Read the model definition and answer for the solid it produces. Units are mm, in the model's axes. A direction names the side the tool comes from. Coordinates: 2 decimals unless noted, no trailing zeros. Order: outer loops, then holes, each group sorted by start corner. A loop starts at its lowest first (then second) coordinate and runs counter-clockwise, first axis right, second up. Notation, with made-up numbers: M 74.5,44 L 103.5,44 A20 ccw 103.5,71 Z; hole C 35,72.5 d2. An arc over 180 degrees is marked long. Put each result on its own line as item: value.
from build123d import *

# Parameters (mm, degrees)
SKETCH1_R                    = 4
BASE_FLANGE1_DEPTH           = 0.8128
EDGE_FLANGE1_STRIP_W         = 4.8768
EDGE_FLANGE1_STRIP_H         = 0.8128
EDGE_FLANGE1_STRIP_CUT_DEPTH = 50
EDGE_FLANGE1_DEPTH           = 50
FILLET2_R                    = 2
F_5_0MM_DOWEL_HOLE1_D        = 5


# Sheet-metal steps are written as plain solids
with BuildPart() as part:
    # Sketch1 → Base-Flange1 (new body)
    with BuildSketch(Plane.XY):
        with BuildLine():
            Line((-25, 0), (25, 0))
            Line((25, 0), (25, 5.5))
            ThreePointArc((25, 5.5), (24.414213562, 6.914213562), (23, 7.5))
            Line((23, 7.5), (10, 7.5))
            ThreePointArc((10, 7.5), (8.585786438, 8.085786438), (8, 9.5))
            Line((8, 9.5), (8, 13.64))
            ThreePointArc((8, 13.64), (0, 21.64), (-8, 13.64))
            Line((-8, 13.64), (-8, 9.5))
            ThreePointArc((-8, 9.5), (-8.585786438, 8.085786438), (-10, 7.5))
            Line((-10, 7.5), (-23, 7.5))
            ThreePointArc((-23, 7.5), (-24.414213562, 6.914213562), (-25, 5.5))
            Line((-25, 5.5), (-25, 0))
        make_face()
        with Locations((0, 13.64)):
            Circle(SKETCH1_R, mode=Mode.SUBTRACT)
    extrude(amount=-BASE_FLANGE1_DEPTH)

    # Edge-Flange1 strip (across the edge) → Edge-Flange1 strip cut (cut)
    with BuildSketch(Plane(origin=(25, 0, -0.8128), x_dir=(0, 1, 0), z_dir=(-1, 0, 0))):
        with Locations((-1.6256, -0.4064)):
            Rectangle(EDGE_FLANGE1_STRIP_W, EDGE_FLANGE1_STRIP_H)
    extrude(amount=EDGE_FLANGE1_STRIP_CUT_DEPTH, mode=Mode.SUBTRACT)

    # Edge-Flange1 section (across the edge) → Edge-Flange1 (add)
    with BuildSketch(Plane(origin=(25, 0, -0.8128), x_dir=(0, 1, 0), z_dir=(-1, 0, 0))):
        with BuildLine():
            Line((-0.8128, 0.8128), (-0.8128, 9.1872))
            Line((-0.8128, 9.1872), (0, 9.1872))
            Line((0, 9.1872), (0, 0.8128))
            ThreePointArc((0, 0.8128), (0.238063608, 0.238063608), (0.8128, 0))
            Line((0.8128, 0), (0.8128, -0.8128))
            ThreePointArc((0.8128, -0.8128), (-0.336672783, -0.336672783), (-0.8128, 0.8128))
        make_face()
    extrude(amount=EDGE_FLANGE1_DEPTH)

    # Fillet2
    fillet2_edges = [part.edges().sort_by_distance(p)[0] for p in [
        (25, -0.4064, -10),
        (-25, -0.4064, -10),
    ]]
    fillet(fillet2_edges, radius=FILLET2_R)

    # Ø5.0mm Dowel Hole1 (through all)
    with Locations(Plane(origin=(0, 0, 0), x_dir=(1, 0, 0), z_dir=(0, 1, 0))):
        with Locations((-12.5, 5.8128), (12.5, 5.8128)):
            Hole(F_5_0MM_DOWEL_HOLE1_D / 2)


solid = part.part
Q1. A tool of negligible diameter and unlimited length cuts with its end or side. For faces 5 (the face through (-25, -0.2, -2.5)), 6 (the face through (0, 7, -0.813)), from which of +Z, -Z, +X, -X, +Y, -Y can it reach the whole face along a straight path? Write none if from no direction.
Answers below:
face 5: +Z, -Z, -X, +Y, -Y
face 6: -Z, +X, -X, +Y
Q2. Given pin 1 (2 mm diameter, centred on x = 1.5, z = -2, fed in from +Y); pin 2 (10.5 mm diameter, centred on x = 0, y = 13.64, fed in from +Z); pin 3 (10.5 mm diameter, centred on x = 1.5, y = 14, fed in from -Z); pin 4 (3 mm diameter, centred on y = 15, z = -2.5, fed in from -X), each flat-ended and moving along its own axis, determine where each tip first touches the part or whether it passes through.
Answers below:
pin 1: stops at y = 0.29
pin 2: stops at z = 0
pin 3: stops at z = -0.81
pin 4: passes through
Q3. For a pull along Y with two mould halves and no side action, classify faces 1 (the face through (0, -0.813, -6)), 2 (the face through (0, 0, -6)), 3 (the face through (-10, -0.4, -5.9)), 4 (the face through (-0.867, 9.735, -0.401)) as +Y half, -Y half, draft (parallel to the pull), parting line (faces both ways), or undercut.
Answers below:
face 1: -Y half
face 2: +Y half
face 3: draft
face 4: undercut
Q4. Find section C-C on x = -19.5. Write down the section's boundary in (y, z), plus the area to 3 significant figures.
Answers below:
outline: M -0.81,-10 L 0,-10 L 0,-1.63 A0.81 cw 0.81,-0.81 L 7.5,-0.81 L 7.5,0 L 0.81,0 A1.63 ccw -0.81,-1.63 Z
area: 13.8 mm^2
Q5. Find section B-B on z = -7.5. Write down the section's boundary in (x, y).
Answers below:
outline: M -25,-0.81 L -14.34,-0.81 L -14.34,0 L -25,0 Z; M -10.66,-0.81 L 10.66,-0.81 L 10.66,0 L -10.66,0 Z; M 14.34,-0.81 L 25,-0.81 L 25,0 L 14.34,0 Z
Q6. Consider line 1 along Y through (x, z) = (9, -5); line 2 along Y through (x, z) = (0, -0.2). Determine where each line is inside the solid, lowest interval first.
Answers below:
line 1: y = -0.81 to 0
line 2: y = 0.03 to 9.64, 17.64 to 21.64
Q7. Find section D-D on x = 0. Write down the section's boundary in (y, z), plus the area to 3 significant figures.
Answers below:
outline: M -0.81,-10 L 0,-10 L 0,-1.63 A0.81 cw 0.81,-0.81 L 9.64,-0.81 L 9.64,0 L 0.81,0 A1.63 ccw -0.81,-1.63 Z; M 17.64,-0.81 L 21.64,-0.81 L 21.64,0 L 17.64,0 Z
area: 18.8 mm^2
Q8. Find section A-A on x = -12.5. Write down the section's boundary in (y, z), plus the area to 3 significant figures.
Answers below:
outline: M -0.81,-10 L 0,-10 L 0,-8.31 L -0.81,-8.31 Z; M -0.81,-3.31 L 0,-3.31 L 0,-1.63 A0.81 cw 0.81,-0.81 L 7.5,-0.81 L 7.5,0 L 0.81,0 A1.63 ccw -0.81,-1.63 Z
area: 9.73 mm^2
